Geometry check sheet. Reference: the model listing, model coordinates, mm. Face numbers are marked on the shaded views. A direction names the side the tool comes from. Round coordinates to 2 decimals unless told otherwise and drop trailing zeros. Loops run counter-clockwise (first coordinate to the right, second up) from the corner with the lowest first, then second, coordinate; pieces in that order, holes last.
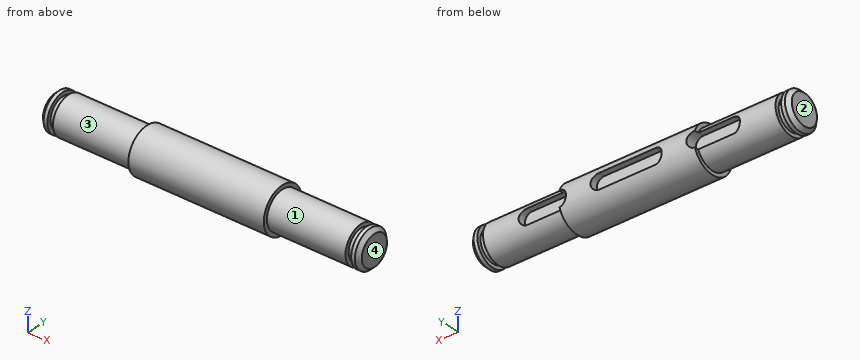
```python
from build123d import *

# Parameters (mm, degrees)
CHAMFER1_SIZE       = 1
SKETCH3_W           = 4
SKETCH3_H           = 4
CUT_EXTRUDE1_DEPTH  = 5
CUT_EXTRUDE2_DEPTH  = 10
CUT_EXTRUDE3_START  = 1
CUT_EXTRUDE3_DEPTH  = 10
BOSS_EXTRUDE1_REACH = 46.071
SKETCH6_W           = 5
SKETCH6_H           = 4


with BuildPart() as part:
    # Sketch1 → Revolve1 (revolve)
    with BuildSketch(Plane.XY, mode=Mode.PRIVATE) as revolve1_sk:
        Polygon((-42.5, 0), (-42.5, 5), (-40.5, 5), (-40.5, 4), (-39, 4), (-39, 5), (-18.05, 5), (-18.05, 6), (18.05, 6), (18.05, 5), (39, 5), (39, 4), (40.5, 4), (40.5, 5), (42.5, 5), (42.5, 0), align=None)
    revolve(revolve1_sk.sketch.rotate(Axis((-47.151991765, 0, 0), (1, 0, 0)), 90), axis=Axis((-47.151991765, 0, 0), (1, 0, 0)))

    # Chamfer1
    chamfer1_edges = [part.edges().sort_by_distance(p)[0] for p in [
        (-42.5, 0, -5),
        (42.5, 0, -5),
    ]]
    chamfer(chamfer1_edges, length=CHAMFER1_SIZE)

    # Sketch3 → Cut-Extrude1 (cut)
    with BuildSketch(Plane(origin=(0, 0, 0), x_dir=(0, 0, -1), z_dir=(1, 0, 0))):
        with Locations((0, 5)):
            Rectangle(SKETCH3_W, SKETCH3_H)
    extrude(amount=-CUT_EXTRUDE1_DEPTH, mode=Mode.SUBTRACT)

    # Sketch4 → Cut-Extrude2 (cut)
    with BuildSketch(Plane(origin=(0, 3, 0), x_dir=(1, 0, 0), z_dir=(0, 1, 0))):
        with BuildLine():
            Line((27.5, -2), (18.05, -2))
            ThreePointArc((18.05, -2), (16.05, 0), (18.05, 2))
            Line((18.05, 2), (27.5, 2))
            ThreePointArc((27.5, 2), (29.5, 0), (27.5, -2))
        make_face()
        with BuildLine():
            Line((-18.05, 2), (-27.5, 2))
            ThreePointArc((-27.5, 2), (-29.5, 0), (-27.5, -2))
            Line((-27.5, -2), (-18.05, -2))
            ThreePointArc((-18.05, -2), (-16.05, 0), (-18.05, 2))
        make_face()
    extrude(amount=CUT_EXTRUDE2_DEPTH, mode=Mode.SUBTRACT)

    # Sketch5 → Cut-Extrude3 (cut)
    with BuildSketch(Plane(origin=(0, 3, 0), x_dir=(1, 0, 0), z_dir=(0, 1, 0)).offset(CUT_EXTRUDE3_START)):
        with BuildLine():
            Line((7.5, -2), (-7.5, -2))
            ThreePointArc((-7.5, -2), (-9.5, 0), (-7.5, 2))
            Line((-7.5, 2), (7.5, 2))
            ThreePointArc((7.5, 2), (9.5, 0), (7.5, -2))
        make_face()
    extrude(amount=CUT_EXTRUDE3_DEPTH, mode=Mode.SUBTRACT)

    # Sketch6 → Boss-Extrude1 (add, up to next)
    with BuildSketch(Plane(origin=(0, 4, 0), x_dir=(1, 0, 0), z_dir=(0, 1, 0)), mode=Mode.PRIVATE) as boss_extrude1_sk1:
        with Locations((-2.5, 0)):
            Rectangle(SKETCH6_W, SKETCH6_H)
    boss_extrude1_tool1 = extrude(boss_extrude1_sk1.sketch, amount=-BOSS_EXTRUDE1_REACH, mode=Mode.PRIVATE) - part.part
    add(boss_extrude1_tool1.solids().sort_by_distance((-2.5, 4, 0))[0])


solid = part.part
```
1) Access from +Z, -Z, +X, -X, +Y, -Y to the whole of each face (thin tool, end or side, straight path). Record for the marked faces 1 and 2.
Report:
face 1: +X
face 2: +Z, -Z, -X, +Y, -Y
2) Sectioned sample at B-B, the plane x = 32.5. Record the cut outline in (y, z).
Report:
outline: circle Ø10 at (0, 0)
3) Mould release check, pull along Z, two halves, no side actions. Record for the marked faces 3 and 4: +Z half, -Z half, draft (parallel to the pull), parting line (faces both ways), or undercut.
Report:
face 3: parting line
face 4: draft
4) Sectioned sample at C-C, the plane x = 23. Record the cut outline in (y, z), then the cut area to 3 significant figures.
Report:
outline: (3, -2) - (3, 2) - (4.58, 2) arc R5 ccw (long way) to (4.58, -2) - close
area: 71.1 mm2
5) Sectioned sample at D-D, the plane x = -6. Record the cut outline in (y, z), then the cut area to 3 significant figures.
Report:
outline: (4, -2) - (4, 2) - (5.66, 2) arc R6 ccw (long way) to (5.66, -2) - close
area: 106 mm2
6) Gauge pin test, flat ends, axial feed: pin 1 (1.3 mm diameter, centred on x = 20.5, y = 3.5, fed in from +Z); pin 2 (4 mm diameter, centred on x = 13.5, y = 3.5, fed in from +Z); pin 3 (3 mm diameter, centred on x = 5.5, z = 1.5, fed in from +Y); pin 4 (5 mm diameter, centred on x = 1.5, z = -1.5, fed in from -Y). Record the tip position at first contact, or that the pin passes through.
Report:
pin 1: stops at z = 4.11
pin 2: stops at z = 5.81
pin 3: stops at y = 5.66
pin 4: stops at y = -6
7) Scan lines: line 1 along X through (y, z) = (4.5, -0.5); line 2 along Z through (x, y) = (22.5, 4); line 3 along Z through (x, y) = (3, 4.5). Record each from-to range of solid material in increasing order.
Report:
line 1: x = -41.97 to -40.5, -39 to -29.44, -16.11 to -9.44, 9.44 to 16.11, 29.44 to 39, 40.5 to 41.97
line 2: z = -3 to -2, 2 to 3
line 3: z = -3.97 to -2, 2 to 3.97
